from build123d import *

# Parameters (mm, degrees)
F0_R         = 12.125
F0_R_2       = 2.5
F1_DEPTH     = 2.38
F2_R         = 12.125
F3_DEPTH     = 1.3
F4_T4_DEPTH  = 25.2617303144
F4_T10_DEPTH = 18.811479046
F4_T15_DEPTH = 18.5490461255
F4_T20_DEPTH = 24.8150280867
F5_R         = 2.5
F6_DEPTH     = 25


# Not quite as in the source:
# - a fillet or chamfer that OpenCascade refuses, or shapes differently, is made with other operations: its cross-section is extruded or revolved along the edge and cut away or added


with BuildPart() as f1:
    # F0 (on Top) → F1 (new body)
    with BuildSketch(Plane.XY):
        Circle(F0_R)
        with Locations((-6.9000022486, 0)):
            Circle(F0_R_2, mode=Mode.SUBTRACT)
        Polygon((-6.9049564988, -9.6863286317), (-6.9049564988, -5.3536104666), (5.4957817031, -0.2610715792), (-6.9049564988, 5.4868851832), (-6.9049564988, 9.8370038228), (11.0929343528, 0.8467586343), (11.0929343528, -1.7459120749), align=None, mode=Mode.SUBTRACT)
    extrude(amount=F1_DEPTH)

    # F2 (on Top) → F3 (join)
    with BuildSketch(Plane.XY):
        Circle(F2_R)
    extrude(amount=F3_DEPTH)

    # F4: chamfer of 1 on 4 edges, made by hand


with BuildPart() as f4_tool2:
    # F4_s3 → F4_t4 (new body)
    with BuildSketch(Plane(origin=(-11.7592465012, 5.8739387937, 0), x_dir=(0, 0, 1), z_dir=(0.8946001051, -0.4468676, 0))):
        Polygon((2.38, -6.7145833148), (1.38, -5.7145833148), (2.38, -5.7145833148), align=None)
    extrude(amount=F4_T4_DEPTH)

    split(bisect_by=Plane.YZ.offset(11.0929343528), keep=Keep.BOTTOM)

    split(bisect_by=Plane.YZ.offset(-6.9049564988), keep=Keep.TOP)


with BuildPart() as f1_1:
    add(f1.part)

    # F4_t1: cut F4_tool2
    add(f4_tool2.part, mode=Mode.SUBTRACT)


with BuildPart() as f4_tool8:
    # F4_s9 → F4_t10 (new body)
    with BuildSketch(Plane(origin=(6.9566759614, -3.2245396996, 0), x_dir=(0, 0, 1), z_dir=(-0.907275067, 0.4205376948, 0))):
        Polygon((2.38, 1.0743196339), (1.38, 2.0743196339), (2.38, 2.0743196339), align=None)
    extrude(amount=F4_T10_DEPTH)

    split(bisect_by=Plane.YZ.offset(-6.9049564988), keep=Keep.TOP)


with BuildPart() as f1_2:
    add(f1_1.part)

    # F4_t7: cut F4_tool8
    add(f4_tool8.part, mode=Mode.SUBTRACT)


with BuildPart() as f4_tool13:
    # F4_s14 → F4_t15 (new body)
    with BuildSketch(Plane(origin=(-10.1686835399, -4.1759140075, 0), x_dir=(0, 0, 1), z_dir=(0.9250361088, 0.3798791878, 0))):
        Polygon((2.38, 1.3292337276), (1.38, 2.3292337276), (2.38, 2.3292337276), align=None)
    extrude(amount=F4_T15_DEPTH)

    split(bisect_by=Plane.YZ.offset(-6.9049564988), keep=Keep.TOP)


with BuildPart() as f1_3:
    add(f1_2.part)

    # F4_t12: cut F4_tool13
    add(f4_tool13.part, mode=Mode.SUBTRACT)


with BuildPart() as f4_tool18:
    # F4_s19 → F4_t20 (new body)
    with BuildSketch(Plane(origin=(10.9936482118, 4.8502431202, 0), x_dir=(0, 0, 1), z_dir=(-0.914914599, -0.4036474657, 0))):
        Polygon((2.38, -7.0749952843), (1.38, -6.0749952843), (2.38, -6.0749952843), align=None)
    extrude(amount=F4_T20_DEPTH)

    split(bisect_by=Plane.YZ.offset(11.0929343528), keep=Keep.BOTTOM)

    split(bisect_by=Plane.YZ.offset(-6.9049564988), keep=Keep.TOP)


with BuildPart() as f1_4:
    add(f1_3.part)

    # F4_t17: cut F4_tool18
    add(f4_tool18.part, mode=Mode.SUBTRACT)

    # F5 (on face) → F6 (cut)
    with BuildSketch(Plane.XY.offset(2.38)):
        with Locations((-6.9000022486, 0)):
            Circle(F5_R)
    extrude(amount=-F6_DEPTH, mode=Mode.SUBTRACT)


solid = f1_4.part
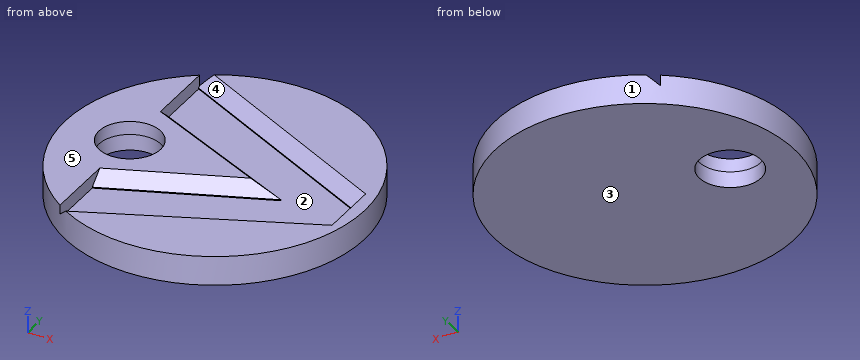
The model under review builds one solid part; all positions refer to its coordinate system, in mm. Face numbers are marked on the shaded views. A direction names the side the tool comes from. Round coordinates to 2 decimals unless told otherwise and drop trailing zeros. Order: outer loops, then holes, each group sorted by start corner. A loop starts at its lowest first (then second) coordinate and runs counter-clockwise, first axis right, second up. Notation, with made-up numbers: (10.25, 54.5) -> (61.25, 54.5) arc R19 cw to (61.25, 79.5) -> close; hole circle Ø8 at (-28.75, 75). An arc over 180 degrees is marked (long way). Write item = value, one per line. Start each with the question number.
Item 1: Consider section C-C on y = 6.25. Write out the cut boundary in (x, z), plus the area to 3 significant figures.
Item 2: Consider section D-D on x = 6.25. Write out the cut boundary in (y, z), plus the area to 3 significant figures.
Item 3: For line 1 along X through (y, z) = (0, 0.1) (3 decimals); line 2 along X through (y, z) = (1, 1.4); line 3 along Y through (x, z) = (-4.25, 1.7), list the stretches that pass through material, from the lowest coordinate up.
Item 4: Consider section B-B on x = -5.5. Write out the cut boundary in (y, z).
Item 5: Mouldability with a two-part tool opening along Y and no side actions: class the marked faces 1, 2 and 3 as released by +Y, released by -Y, zero draft, split by the parting line, or undercut.
Item 6: Consider section A-A on z = 1.95. Write out the cut boundary in (x, y) (3 decimals).
Item 7: For the marked faces 4 and 5, list the 3-axis set-ups (+Z, -Z, +X, -X, +Y, -Y) from which the entire face can be reached by the end or side of a thin tool; tool diameter is ignored.
Item 8: Clearance check with flat-ended pins moving along their axes: pin 1 Ø1 at (x, y) = (-0.5, -6) entering from +Z; pin 2 Ø0.5 at (y, z) = (-8.5, 2) entering from +X; pin 3 Ø0.5 at (y, z) = (7, 2) entering from +X; pin 4 Ø4.5 at (x, y) = (-6.9, 0) entering from -Z. State where each tip first meets the part, or that it passes through.
Conclusion:
q1.outline = (-10.39, 0) -> (10.39, 0) -> (10.39, 2.38) -> (2.51, 2.38) -> (0.28, 1.38) -> (0.28, 1.3) -> (-6.9, 1.3) -> (-6.9, 2.38) -> (-10.39, 2.38) -> close
q1.area = 40.6 mm2
q2.outline = (-10.39, 0) -> (10.39, 0) -> (10.39, 2.38) -> (4.38, 2.38) -> (3.27, 1.38) -> (3.27, 1.3) -> (-3.88, 1.3) -> (-3.88, 1.38) -> (-4.98, 2.38) -> (-10.39, 2.38) -> close
q2.area = 40.6 mm2
q3.line_1 = -12.125 to -9.4, -4.4 to 12.125
q3.line_2 = -12.08 to -9.19, -4.61 to 2.73, 10.83 to 12.08
q3.line_3 = -11.36 to -8.86, -3.92 to 3.9, 8.87 to 11.36
q4.outline = (-10.81, 0) -> (-2.07, 0) -> (-2.07, 2.38) -> (-3.7, 2.38) -> (-4.78, 1.38) -> (-4.78, 1.3) -> (-9.07, 1.3) -> (-9.07, 1.38) -> (-10.16, 2.38) -> (-10.81, 2.38) -> close; (2.07, 0) -> (10.81, 0) -> (10.81, 2.38) -> (10.25, 2.38) -> (9.14, 1.38) -> (9.14, 1.3) -> (4.84, 1.3) -> (4.84, 1.38) -> (3.73, 2.38) -> (2.07, 2.38) -> close
q5.face_1 = split by the parting line
q5.face_2 = undercut
q5.face_3 = zero draft
q6.outline = (-6.905, -9.967) -> (-6.905, -4.737) -> (4.072, -0.229) -> (-6.905, 4.859) -> (-6.905, 9.967) arc R12.125 ccw to start; (-6.597, -10.173) arc R12.125 ccw (long way) to (-6.468, 10.256) -> (11.093, 1.484) -> (11.093, -2.369) -> close; hole circle Ø5 at (-6.9, 0)
q7.face_4 = +Z
q7.face_5 = +Z, +X, -X, +Y, -Y
q8.pin_1 = 1.3
q8.pin_2 = 8.89
q8.pin_3 = 10.07
q8.pin_4 = through
